Drawing for the job (mm, zero at the part's lowest x, y, z). Round coordinates to 2 decimals unless told otherwise and drop trailing zeros. Write each loop counter-clockwise with the first axis right and the second up, starting at its lowest first coordinate (ties: lowest second). Pieces come first, ordered by that corner, then holes. Notation, with made-up numbers: M 52.25,0 L 82.25,0 A37 ccw 82.25,37 Z; hole C 54,9.25 d11. An arc over 180 degrees is marked long. Use a Markdown table: item, result.
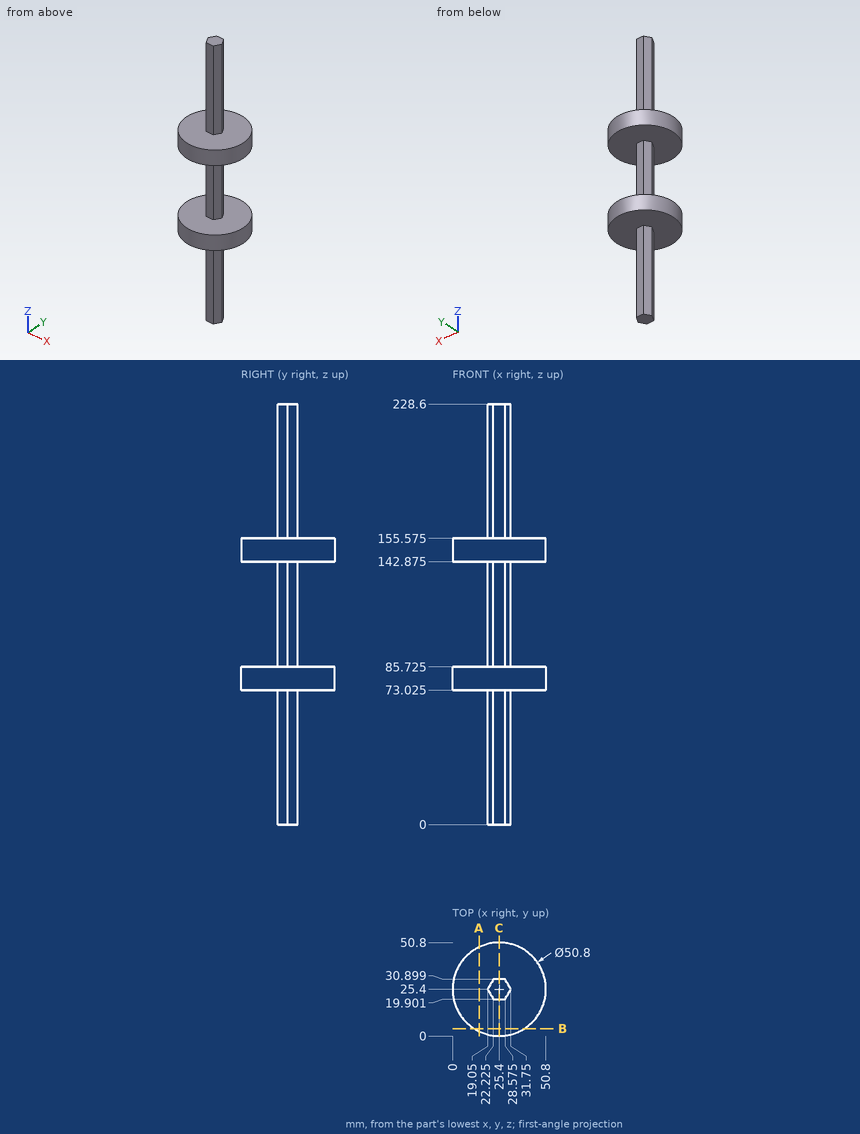
Q1. Cut at B-B on y = 4. Give the cut face in (x, z) (1 decimal).
Response values:
| item | result |
|---|---|
| outline | M 11.7,73 L 39.1,73 L 39.1,85.7 L 11.7,85.7 Z; M 11.7,142.9 L 39.1,142.9 L 39.1,155.6 L 11.7,155.6 Z |
Q2. Cut at C-C on x = 25.4. Give the cut face in (y, z) (1 decimal).
Response values:
| item | result |
|---|---|
| outline | M 0,73 L 19.9,73 L 19.9,0 L 30.9,0 L 30.9,73 L 50.8,73 L 50.8,85.7 L 30.9,85.7 L 30.9,142.9 L 50.8,142.9 L 50.8,155.6 L 30.9,155.6 L 30.9,228.6 L 19.9,228.6 L 19.9,155.6 L 0,155.6 L 0,142.9 L 19.9,142.9 L 19.9,85.7 L 0,85.7 Z |
Q3. Drill centre lines: L1, parallel to Z at x = 13, y = 29.5 (1 decimal); L2, parallel to Y at x = 25.5, z = 84; L3, parallel to Y at x = 22.5, z = 95. Where is each one in solid material? Low to high.
Response values:
| item | result |
|---|---|
| L1 | z = 73 to 85.7, 142.9 to 155.6 |
| L2 | y = 0 to 50.8 |
| L3 | y = 19.9 to 30.9 |
Q4. Cut at A-A on x = 14.5. Give the cut face in (y, z) (1 decimal), and give its area (3 significant figures).
Response values:
| item | result |
|---|---|
| outline | M 2.5,73 L 48.3,73 L 48.3,85.7 L 2.5,85.7 Z; M 2.5,142.9 L 48.3,142.9 L 48.3,155.6 L 2.5,155.6 Z |
| area | 1,170 mm2 |
Q5. Drop flat-ended pins along their axis: P1, Ø1.5, axis at x = 11, y = 38.5, coming from the +Z side (3 decimals); P2, Ø1.5, axis at x = 29.5, z = 102, coming from the +Y side (1 decimal); P3, Ø10, axis at x = 9.5, y = 32, coming from the -Z side (3 decimals). Give the stop position or say it passes through.
Response values:
| item | result |
|---|---|
| P1 | stops at z = 155.575 |
| P2 | stops at y = 30.6 |
| P3 | stops at z = 73.025 |
